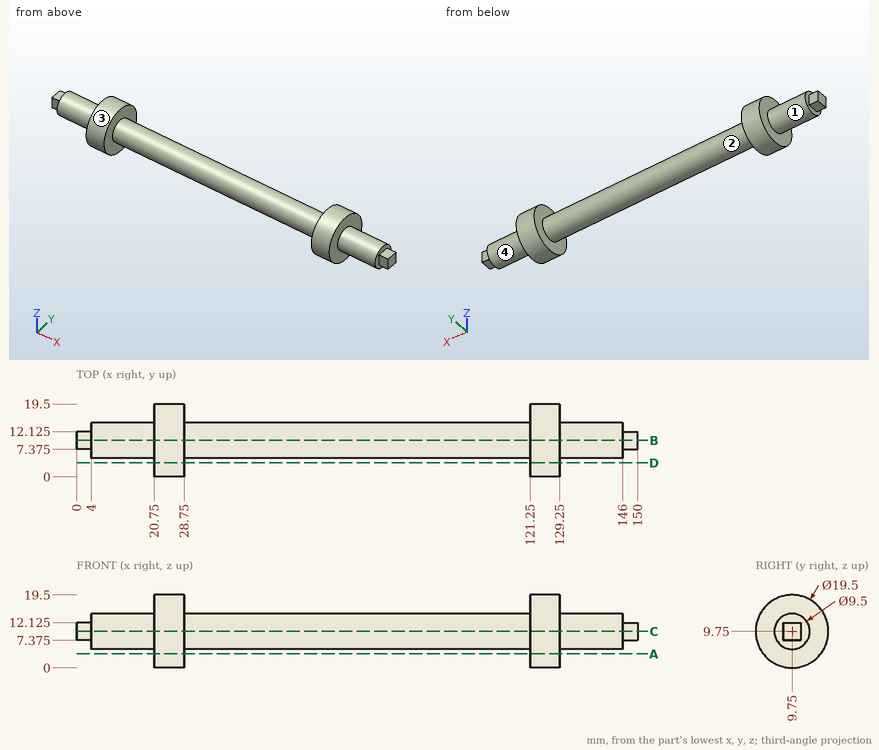
Geometry: see drawing. Coordinates: mm, zero at the bounding-box minimum. A direction names the side the tool comes from. Round coordinates to 2 decimals unless told otherwise and drop trailing zeros. Write each loop counter-clockwise with the first axis right and the second up, starting at its lowest first coordinate (ties: lowest second). Pieces come first, ordered by that corner, then holes. Notation, with made-up numbers: M 41.25,58 L 47.25,58 A16 ccw 47.25,84 Z; hole C 21,42 d6. An arc over 180 degrees is marked long. Answer in a Markdown table with one row per item. Add a question column.
(1) Draft query along X for the marked faces 1 and 2. Return one class per face: pulls with the +X half, pulls with the -X half, needs draft (parallel to the pull), parting line crosses it, or undercut.
(2) Contact query for flat-ended pins moving along their axis: pin 1 (8 mm diameter, centred on x = 117.5, z = 14.5, fed in from -Y); pin 2 (1.2 mm diameter, centred on x = 2, y = 9.5, fed in from +Z) (3 decimals); pin 3 (4.5 mm diameter, centred on x = 1, z = 10, fed in from +Y) (3 decimals); pin 4 (5 mm diameter, centred on x = 39.5, y = 2, fed in from +Z). Output: stop coordinate, or through.
(3) Cut plane B-B, the plane y = 9.75. Return the cut outline in (x, z) (3 decimals).
(4) Reachability of the marked faces 3 and 4 from +Z, -Z, +X, -X, +Y, -Y: full face, straight path, thin tool, end or side. Return the list, or none.
(5) Cut plane A-A, the plane z = 3.75. Return the cut outline in (x, y).
(6) Ray query, L1, parallel to X at y = 4.5, z = 16; L2, parallel to Y at x = 9, z = 9.5; L3, parallel to X at y = 12.5, z = 13. Return the intervals inside material, ascending.
Established:
| question | item | result |
|---|---|---|
| 1 | face 1 | needs draft |
| 1 | face 2 | undercut |
| 2 | pin 1 | y = 0.6 |
| 2 | pin 2 | z = 12.125 |
| 2 | pin 3 | y = 12.125 |
| 2 | pin 4 | through |
| 3 | outline | M 0,7.375 L 4,7.375 L 4,5 L 20.75,5 L 20.75,0 L 28.75,0 L 28.75,5 L 121.25,5 L 121.25,0 L 129.25,0 L 129.25,5 L 146,5 L 146,7.375 L 150,7.375 L 150,12.125 L 146,12.125 L 146,14.5 L 129.25,14.5 L 129.25,19.5 L 121.25,19.5 L 121.25,14.5 L 28.75,14.5 L 28.75,19.5 L 20.75,19.5 L 20.75,14.5 L 4,14.5 L 4,12.125 L 0,12.125 Z |
| 4 | face 3 | +X, -X |
| 4 | face 4 | +X |
| 5 | outline | M 20.75,2.06 L 28.75,2.06 L 28.75,17.44 L 20.75,17.44 Z; M 121.25,2.06 L 129.25,2.06 L 129.25,17.44 L 121.25,17.44 Z |
| 6 | L1 | 20.75 to 28.75, 121.25 to 129.25 |
| 6 | L2 | 5.01 to 14.49 |
| 6 | L3 | 4 to 146 |
